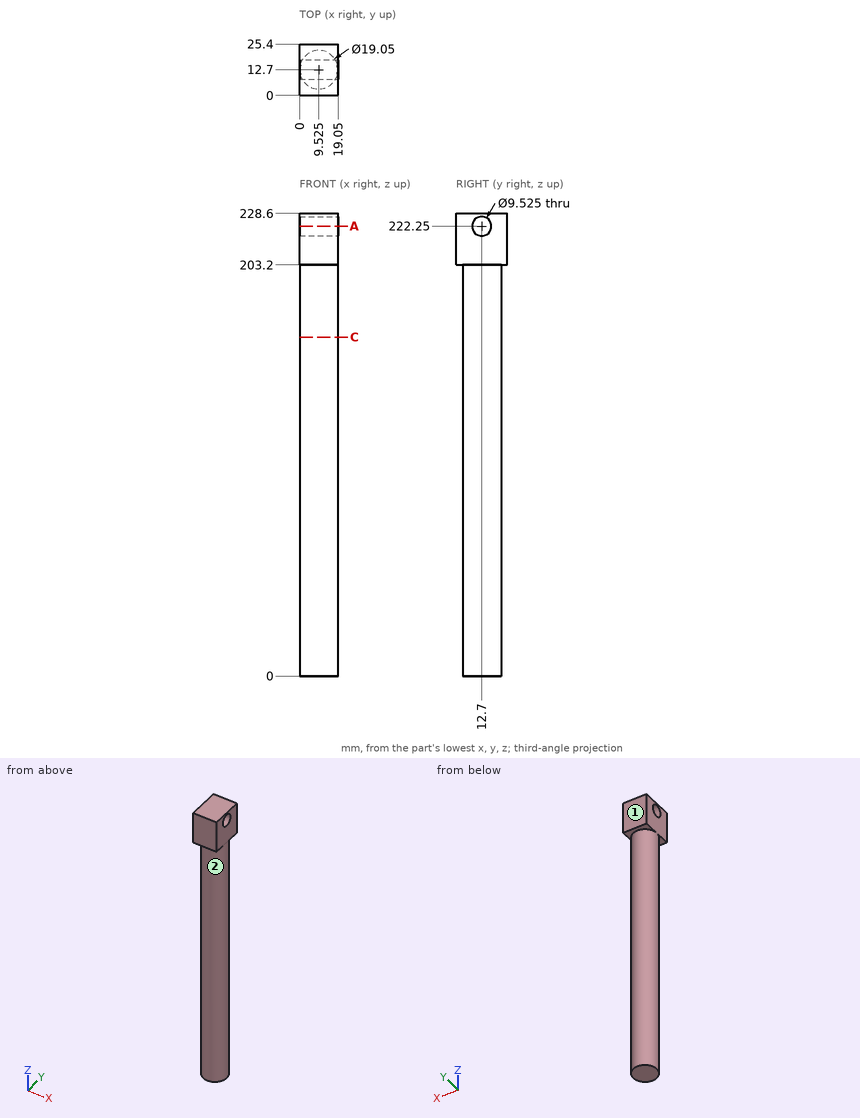
Answer from the drawing. Dimensions are ordinates in mm from the lowest x, y and z of the part. A direction names the side the tool comes from. Give positions to 0.01 mm unless a question says otherwise; leave off trailing zeros. Order: outer loops, then holes, each group sorted by start corner. A loop starts at its lowest first (then second) coordinate and runs counter-clockwise, first axis right, second up. Notation, with made-up numbers: (-6, 47) - (36, 47) arc R26 cw to (36, 76) - close; hole circle Ø9 at (1.25, 82.25). An arc over 180 degrees is marked (long way). Use one line per item in the form item = value.
1) Consider probe 1 along Z at (x, y) = (5.75, 12.7); probe 2 along Z at (x, y) = (13.25, 16); probe 3 along X at (y, z) = (13.25, 53.5). Determine where each line is inside the solid, lowest interval first. Write a range as [from, to].
Verdict:
probe_1 = [0, 217.49], [227.01, 228.6]
probe_2 = [0, 218.82], [225.68, 228.6]
probe_3 = [0.02, 19.03]
2) For the marked faces 1 and 2, determine the directions among +Z, -Z, +X, -X, +Y, -Y from which every point of the face is accessible in a straight line to the end or side of a thin tool.
Verdict:
face_1 = +Z, -Z, +X, -X, +Y
face_2 = -Z
3) Find section C-C on z = 167.5. Determine the outline of the cut face in (x, y) (3 decimals), and give its area (3 significant figures).
Verdict:
outline = circle Ø19.05 at (9.525, 12.7)
area = 285 mm^2
4) Find section A-A on z = 222.25. Determine the outline of the cut face in (x, y).
Verdict:
outline = (0, 0) - (19.05, 0) - (19.05, 7.94) - (0, 7.94) - close; (0, 17.46) - (19.05, 17.46) - (19.05, 25.4) - (0, 25.4) - close
5) Each of these flat-tipped pins is pushed along its axis until it touches: pin 1 (4 mm diameter, centred on x = 10, z = 26, fed in from -Y) (3 decimals); pin 2 (4 mm diameter, centred on x = 6, z = 29, fed in from +Y); pin 3 (8 mm diameter, centred on y = 17.5, z = 118, fed in from -X). Where does it stop, or does it pass through?
Verdict:
pin_1 = 3.175
pin_2 = 22.1
pin_3 = 0.03
